The model under review builds one solid part; all positions refer to its coordinate system, in mm. A direction names the side the tool comes from. Give positions to 0.01 mm unless a question says otherwise; leave off trailing zeros. Loops run counter-clockwise (first coordinate to the right, second up) from the corner with the lowest first, then second, coordinate; pieces in that order, holes last. Notation, with made-up numbers: M 58.5,36 L 72.5,36 A16 cw 72.5,62 Z; hole C 47.25,-5.75 d11. An arc over 180 degrees is marked long. Write item = value, one per line. Start each with the question number.
1. We need section B-B on z = 78.5. Count the separate pieces of the cut face and the enclosed holes in it, then the cut area to 3 significant figures.
2. Wall thickness on line 1 along X through (y, z) = (-2.75, -18); line 2 along Y through (x, z) = (-8.75, 98); line 3 along X through (y, z) = (4.25, -28): over which ranges is each line inside the solid? List them lowest first. Write a range as from..to.
3. For faces 4 (the face through (0, -1.702, 58)), 5 (the face through (5.513, 0.83, 58.484)), 6 (the face through (8, -6.35, 58)), list the 3-axis set-ups (+Z, -Z, +X, -X, +Y, -Y) from which the entire face can be reached by the end or side of a thin tool; tool diameter is ignored.
4. We need section A-A on x = 0. Give the boundary of the cut face in (y, z), then the cut area to 3 significant figures.
5. Draft analysis for pull direction X (two halves, no side actions). For faces 1 (the face through (0, -3, 152.4)), 2 (the face through (-12.7, 0, 58)), 3 (the face through (10.337, -1.151, 55.817)), state which applies: pulls with the +X half, pulls with the -X half, needs draft (parallel to the pull), parting line crosses it, or undercut.
6. For pin 1 (2.5 mm diameter, centred on x = 8.72, y = -2.39, fed in from -Z); pin 2 (1 mm diameter, centred on x = -3, z = 128, fed in from +Y); pin 3 (3 mm diameter, centred on x = 0, z = 31, fed in from +Y), all flat-tipped, find the tip position at first contact; note any pin that passes through.
from build123d import *

# Parameters (mm, degrees)
SKETCH3_R               = 2.032
BOSS_EXTRUDE1_DEPTH     = 152.4
CUT_EXTRUDE1_DEPTH      = 154.060029074
CUT_EXTRUDE1_DEPTH_BACK = 154.060029074
SKETCH4_R               = 0.55245
SKETCH5_W               = 50.8
SKETCH5_H               = 114.3
CUT_EXTRUDE2_DEPTH      = 154.454683865


with BuildPart() as part:
    # Sketch3 → Boss-Extrude1 (new, symmetric)
    with BuildSketch(Plane.XY):
        with BuildLine():
            Line((3.2512, 5.35559), (3.2512, 5.13461))
            ThreePointArc((3.2512, 5.13461), (3.542455946, 4.431455946), (4.24561, 4.1402))
            Line((4.24561, 4.1402), (6.42239, 4.1402))
            ThreePointArc((6.42239, 4.1402), (7.341105046, 3.526334232), (7.125544054, 2.442635946))
            Line((7.125544054, 2.442635946), (3.854875946, -0.828032163))
            ThreePointArc((3.854875946, -0.828032163), (2.887046479, -1.474715138), (1.745413783, -1.7018))
            Line((1.745413783, -1.7018), (0, -1.7018))
            Line((0, -1.7018), (0, -6.35))
            Line((0, -6.35), (10.16, -6.35))
            ThreePointArc((10.16, -6.35), (11.956051224, -5.606051224), (12.7, -3.81))
            Line((12.7, -3.81), (12.7, 3.81))
            ThreePointArc((12.7, 3.81), (11.956051224, 5.606051224), (10.16, 6.35))
            Line((10.16, 6.35), (4.24561, 6.35))
            ThreePointArc((4.24561, 6.35), (3.542455946, 6.058744054), (3.2512, 5.35559))
        make_face()
        with Locations(Location((8.7249, -2.3876, 0), (0, 0, 180))):
            Circle(SKETCH3_R, mode=Mode.SUBTRACT)
    extrude(amount=BOSS_EXTRUDE1_DEPTH, both=True)

    # Sketch4 → Cut-Extrude1 (cut, two sides: drawn at the far end of the back side and taken through both)
    with BuildSketch(Plane.XY.offset(-CUT_EXTRUDE1_DEPTH_BACK)):
        with Locations((5.86994, 6.35)):
            Circle(SKETCH4_R)
        with Locations((10.20445, 6.35)):
            Circle(SKETCH4_R)
        with Locations((5.86994, -6.35)):
            Circle(SKETCH4_R)
        with Locations((10.20445, -6.35)):
            Circle(SKETCH4_R)
    extrude(amount=CUT_EXTRUDE1_DEPTH + CUT_EXTRUDE1_DEPTH_BACK, mode=Mode.SUBTRACT)

    # Mirror1: part across plane


with BuildPart() as part_1:
    add(part.part)
    add(part.part.mirror(Plane(origin=(0, 0, 0), x_dir=(0, 0, 1), z_dir=(1, 0, 0))))

    # Sketch5 → Cut-Extrude2 (cut, through all)
    with BuildSketch(Plane.XZ.offset(6.35)):
        with Locations((0, -95.25)):
            Rectangle(SKETCH5_W, SKETCH5_H)
    extrude(amount=-CUT_EXTRUDE2_DEPTH, mode=Mode.SUBTRACT)


solid = part_1.part
Final values:
q1.separate_pieces = 1
q1.enclosed_holes = 2
q1.area = 206 mm²
q2.line_1 = -12.7..-10.72, -6.73..6.73, 10.72..12.7
q2.line_2 = -6.35..-4.42, -0.36..6.35
q2.line_3 = -12.66..-3.79, 3.79..12.66
q3.face_4 = +Z, -Z, +Y
q3.face_5 = +Z, -Z
q3.face_6 = +Z, -Z, +X, -X, -Y
q4.outline = M -6.35,-38.1 L -1.7,-38.1 L -1.7,152.4 L -6.35,152.4 Z
q4.area = 885 mm²
q5.face_1 = needs draft
q5.face_2 = pulls with the -X half
q5.face_3 = undercut
q6.pin_1 = through
q6.pin_2 = 6.01
q6.pin_3 = -1.7
